Read the model definition and answer for the solid it produces. Units are mm, in the model's axes. A direction names the side the tool comes from. Give positions to 0.01 mm unless a question says otherwise; leave off trailing zeros. Write each loop counter-clockwise with the first axis right and the second up, starting at its lowest first coordinate (ties: lowest second). Pieces come first, ordered by that corner, then holes. Notation, with made-up numbers: M 58,51.5 L 112,51.5 A20 cw 112,57.5 Z; hole C 0.25,-13 d9. An arc over 180 degrees is marked long. Use a Markdown table: item, result. Add a question column.
Item 1: A cutting plane is placed at D-D on y = 51.5. Determine the outline of the cut face in (x, z).
Item 2: A cutting plane is placed at B-B on y = 81.75. Determine the outline of the cut face in (x, z), then the cut area to 3 significant figures.
Item 3: A cutting plane is placed at A-A on y = -17. Determine the outline of the cut face in (x, z).
Item 4: Given P1, Ø5, axis at y = -107.5, z = 0, coming from the +X side; P2, Ø5, axis at x = 14, z = 2.5, coming from the -Y side; P3, Ø3, axis at y = 52, z = -1, coming from the +X side; P4, Ø8, axis at x = -21, y = 83.5, coming from the -Z side, each flat-ended and moving along its own axis, determine where each tip first touches the part or whether it passes through.
Item 5: The mould has two halves that part along Y. Classify faces 1 (the cylindrical face through (23.4, -92.82, 0.07)), 2 (the cylindrical face through (-21.71, 78.47, -2.54)), 3 (the flat face through (0, -1, 5)), 4 (the flat face through (-12, -89.25, 0)): pulls with the +Y half, pulls with the -Y half, needs draft (parallel to the pull), parting line crosses it, or undercut.
Item 6: A cutting plane is placed at C-C on x = 2. Determine the outline of the cut face in (y, z).
Item 7: Consider probe 1 along X at (y, z) = (17.5, 2.25); probe 2 along X at (y, z) = (68, -3.25); probe 3 along X at (y, z) = (82, 1.25). Determine where each line is inside the solid, lowest interval first. Write a range as [from, to].
Item 8: For faces 5 (the flat face through (-20.01, 54.03, -0.07)), 6 (the flat face through (-15, -115, 0)), 7 (the flat face through (18, 80, 0)), 8 (the flat face through (-5, -45, 0)), 9 (the flat face through (19.89, -53.82, -0.07)), determine the directions among +Z, -Z, +X, -X, +Y, -Y from which every point of the face is accessible in a straight line to the end or side of a thin tool.
from build123d import *

# Parameters (mm, degrees)
SKETCH_1_W          = 49.8
SKETCH_1_H          = 188.5
EXTRUDE_1_DEPTH     = 5
CUT_EXTRUDE_1_DEPTH = 98.995267743
FILLET_1_R          = 5
CUT_EXTRUDE_2_DEPTH = 98.995267743
CHAMFER_2_SIZE      = 20
SKETCH_3_W          = 30
SKETCH_3_H          = 6
EXTRUDE_2_DEPTH     = 48
CHAMFER_3_SIZE      = 5
SKETCH_6_R          = 2.1
CUT_EXTRUDE_6_DEPTH = 145.758669861
SKETCH_7_R          = 3.7
CUT_EXTRUDE_7_DEPTH = 5


with BuildPart() as part:
    # 草图1 → 凸台-拉伸1 (new, symmetric)
    with BuildSketch(Plane.XY):
        Rectangle(SKETCH_1_W, SKETCH_1_H)
    extrude(amount=EXTRUDE_1_DEPTH, both=True)

    # 草图4 → 切除-拉伸1 (cut, through all)
    with BuildSketch(Plane(origin=(0, 0, -5), x_dir=(-1, 0, 0), z_dir=(0, 0, -1))):
        Polygon((-24.9, 62.5), (-15, 45.352697005), (-15, -45.352697005), (-24.9, -62.5), align=None)
        Polygon((24.9, -62.5), (24.9, 62.5), (15, 45.352697005), (15, -45.352697005), align=None)
    extrude(amount=-CUT_EXTRUDE_1_DEPTH, mode=Mode.SUBTRACT)

    # 圆角1
    fillet_1_edges = [part.edges().sort_by_distance(p)[0] for p in [
        (24.9, -62.5, 0),
        (24.9, 62.5, 0),
        (15, 45.352697005, 0),
        (15, -45.352697005, 0),
        (-24.9, -62.5, 0),
        (-15, -45.352697005, 0),
        (-15, 45.352697005, 0),
        (-24.9, 62.5, 0),
        (24.9, -94.25, 0),
        (-24.9, -94.25, 0),
        (-24.9, 94.25, 0),
        (24.9, 94.25, 0),
    ]]
    fillet(fillet_1_edges, radius=FILLET_1_R)

    # 草图5 → 切除-拉伸2 (cut, through all)
    with BuildSketch(Plane(origin=(0, 0, -5), x_dir=(-1, 0, 0), z_dir=(0, 0, -1))):
        Polygon((-19.9, 89.25), (-19.9, 63.839745962), (-10, 46.692442967), (-10, 2.5), (-5, 2.5), (-5, 89.25), align=None)
        Polygon((5, 89.25), (19.9, 89.25), (19.9, 63.839745962), (10, 46.692442967), (10, 2.5), (5, 2.5), align=None)
        Polygon((19.9, -89.25), (19.9, -63.839745962), (10, -46.692442967), (10, -2.5), (5, -2.5), (5, -89.25), align=None)
        Polygon((-5, -89.25), (-19.9, -89.25), (-19.9, -63.839745962), (-10, -46.692442967), (-10, -2.5), (-5, -2.5), align=None)
    extrude(amount=-CUT_EXTRUDE_2_DEPTH, mode=Mode.SUBTRACT)

    # 倒角2
    # the kernel refuses this chamfer: 20 mm, written as the material it adds along each edge
    with BuildSketch(Plane(origin=(-19.9, 89.25, -5), x_dir=(-0.027495876610586317, -0.9996219169112968, 0), z_dir=(0, 0, 1))) as chamfer_2_piece_1:
        Polygon((CHAMFER_2_SIZE * 0.999621916911, CHAMFER_2_SIZE * 0.0274958766106), (-CHAMFER_2_SIZE * 0.0274958766106, CHAMFER_2_SIZE * 0.999621916911), (0, 0), align=None)
    extrude(amount=10)
    with BuildSketch(Plane(origin=(19.9, 89.25, -5), x_dir=(0.027495876610586317, -0.9996219169112968, 0), z_dir=(0, 0, 1))) as chamfer_2_piece_2:
        Polygon((CHAMFER_2_SIZE * 0.999621916911, -CHAMFER_2_SIZE * 0.0274958766106), (-CHAMFER_2_SIZE * 0.0274958766106, -CHAMFER_2_SIZE * 0.999621916911), (0, 0), align=None)
    extrude(amount=10)

    # 草图3 → 凸台-拉伸2 (add)
    with BuildSketch(Plane.XZ.offset(94.25)):
        Rectangle(SKETCH_3_W, SKETCH_3_H)
    extrude(amount=EXTRUDE_2_DEPTH)

    # 倒角3
    chamfer_3_edges = [part.edges().sort_by_distance(p)[0] for p in [
        (15, -142.25, 0),
        (-15, -142.25, 0),
    ]]
    chamfer(chamfer_3_edges, length=CHAMFER_3_SIZE)

    # 草图6 → 切除-拉伸6 (cut, through all)
    with BuildSketch(Plane.XY.offset(5)):
        with Locations((-20, 81.75)):
            Circle(SKETCH_6_R)
        with Locations(Location((20, 81.75, 0), (0, 0, 180))):
            Circle(SKETCH_6_R)
    extrude(amount=-CUT_EXTRUDE_6_DEPTH, mode=Mode.SUBTRACT)

    # 草图7 → 切除-拉伸7 (cut)
    with BuildSketch(Plane(origin=(0, 0, -5), x_dir=(-1, 0, 0), z_dir=(0, 0, -1))):
        with Locations((20, 81.75)):
            Circle(SKETCH_7_R)
        with Locations((-20, 81.75)):
            Circle(SKETCH_7_R)
    extrude(amount=-CUT_EXTRUDE_7_DEPTH, mode=Mode.SUBTRACT)


solid = part.part
Filled in:
| question | item | result |
|---|---|---|
| 1 | outline | M -18.55,-5 L -12.78,-5 L -12.78,5 L -18.55,5 Z; M -5,-5 L 5,-5 L 5,5 L -5,5 Z; M 12.78,-5 L 18.55,-5 L 18.55,5 L 12.78,5 Z |
| 2 | outline | M -24.9,-5 L -23.7,-5 L -23.7,0 L -22.1,0 L -22.1,5 L -24.9,5 Z; M -17.9,0 L -16.3,0 L -16.3,-5 L -7.4,-5 L -7.4,5 L -17.9,5 Z; M -5,-5 L 5,-5 L 5,5 L -5,5 Z; M 7.4,-5 L 16.3,-5 L 16.3,0 L 17.9,0 L 17.9,5 L 7.4,5 Z; M 22.1,0 L 23.7,0 L 23.7,-5 L 24.9,-5 L 24.9,5 L 22.1,5 Z |
| 2 | area | 334 mm² |
| 3 | outline | M -15,-5 L -10,-5 L -10,5 L -15,5 Z; M -5,-5 L 5,-5 L 5,5 L -5,5 Z; M 10,-5 L 15,-5 L 15,5 L 10,5 Z |
| 4 | P1 | x = 15 |
| 4 | P2 | y = -140.75 |
| 4 | P3 | x = 19.7 |
| 4 | P4 | z = -5 |
| 5 | face 1 | pulls with the -Y half |
| 5 | face 2 | undercut |
| 5 | face 3 | needs draft |
| 5 | face 4 | undercut |
| 6 | outline | M -142.25,-3 L -94.25,-3 L -94.25,-5 L 94.25,-5 L 94.25,5 L -94.25,5 L -94.25,3 L -142.25,3 Z |
| 7 | probe 1 | [-15, -10], [-5, 5], [10, 15] |
| 7 | probe 2 | [-24.9, -19.9], [-5, 5], [19.9, 24.9] |
| 7 | probe 3 | [-24.9, -22.09], [-17.91, -7.15], [-5, 5], [7.15, 17.91], [22.09, 24.9] |
| 8 | face 5 | +Z, -Z, -X |
| 8 | face 6 | +Z, -Z, -X, -Y |
| 8 | face 7 | -Z |
| 8 | face 8 | +Z, -Z |
| 8 | face 9 | +Z, -Z, +X |
